Verification items for the finished model (mm, model axes). A direction names the side the tool comes from. Round coordinates to 2 decimals unless told otherwise and drop trailing zeros. Loops run counter-clockwise (first coordinate to the right, second up) from the corner with the lowest first, then second, coordinate; pieces in that order, holes last. Notation, with made-up numbers: (16, 22) - (24, 22) arc R23 ccw to (24, 54) - close; hole circle Ø9 at (13.25, 55.5). An arc over 180 degrees is marked (long way). Use CSV: the item, a comma, the result in double quotes.
```python
from build123d import *

# Parameters (mm, degrees)
F0_R          = 3
F0_R_2        = 2.5
F1_DEPTH      = 115.678
F2_R          = 2
F3_R          = 7
F6_DEPTH      = 30
F6_DEPTH_BACK = 30
F7_W          = 131.1645284295
F7_H          = 50.7057756186
F8_DEPTH      = 30
F8_DEPTH_BACK = 30


# Not quite as in the source:
# - a feature names something its author has since deleted; it is built from what else it names


with BuildPart() as f1:
    # F0 (on Top) → F1 (new body)
    with BuildSketch(Plane.XY):
        with BuildLine():
            Line((18.15, -30), (30, -30))
            Line((30, -30), (30, -18.15))
            Line((30, -18.15), (27.5, -18.15))
            Line((27.5, -18.15), (27.5, -20.15))
            Line((27.5, -20.15), (21.5477069044, -20.15))
            ThreePointArc((21.5477069044, -20.15), (19.5, -15), (21.5477069044, -9.85))
            Line((21.5477069044, -9.85), (27.5, -9.85))
            Line((27.5, -9.85), (27.5, -11.85))
            Line((27.5, -11.85), (30, -11.85))
            Line((30, -11.85), (30, 11.85))
            Line((30, 11.85), (27.5, 11.85))
            Line((27.5, 11.85), (27.5, 9.85))
            Line((27.5, 9.85), (21.5477069044, 9.85))
            ThreePointArc((21.5477069044, 9.85), (19.5, 15), (21.5477069044, 20.15))
            Line((21.5477069044, 20.15), (27.5, 20.15))
            Line((27.5, 20.15), (27.5, 18.15))
            Line((27.5, 18.15), (30, 18.15))
            Line((30, 18.15), (30, 30))
            Line((30, 30), (18.15, 30))
            Line((18.15, 30), (18.15, 27.5))
            Line((18.15, 27.5), (20.15, 27.5))
            Line((20.15, 27.5), (20.15, 21.5477069044))
            ThreePointArc((20.15, 21.5477069044), (15, 19.5), (9.85, 21.5477069044))
            Line((9.85, 21.5477069044), (9.85, 27.5))
            Line((9.85, 27.5), (11.85, 27.5))
            Line((11.85, 27.5), (11.85, 30))
            Line((11.85, 30), (-11.85, 30))
            Line((-11.85, 30), (-11.85, 27.5))
            Line((-11.85, 27.5), (-9.85, 27.5))
            Line((-9.85, 27.5), (-9.85, 21.5477069044))
            ThreePointArc((-9.85, 21.5477069044), (-15, 19.5), (-20.15, 21.5477069044))
            Line((-20.15, 21.5477069044), (-20.15, 27.5))
            Line((-20.15, 27.5), (-18.15, 27.5))
            Line((-18.15, 27.5), (-18.15, 30))
            Line((-18.15, 30), (-30, 30))
            Line((-30, 30), (-30, 18.15))
            Line((-30, 18.15), (-27.5, 18.15))
            Line((-27.5, 18.15), (-27.5, 20.15))
            Line((-27.5, 20.15), (-21.5477069044, 20.15))
            ThreePointArc((-21.5477069044, 20.15), (-19.5, 15), (-21.5477069044, 9.85))
            Line((-21.5477069044, 9.85), (-27.5, 9.85))
            Line((-27.5, 9.85), (-27.5, 11.85))
            Line((-27.5, 11.85), (-30, 11.85))
            Line((-30, 11.85), (-30, -11.85))
            Line((-30, -11.85), (-27.5, -11.85))
            Line((-27.5, -11.85), (-27.5, -9.85))
            Line((-27.5, -9.85), (-21.5477069044, -9.85))
            ThreePointArc((-21.5477069044, -9.85), (-19.5, -15), (-21.5477069044, -20.15))
            Line((-21.5477069044, -20.15), (-27.5, -20.15))
            Line((-27.5, -20.15), (-27.5, -18.15))
            Line((-27.5, -18.15), (-30, -18.15))
            Line((-30, -18.15), (-30, -30))
            Line((-30, -30), (-18.15, -30))
            Line((-18.15, -30), (-18.15, -27.5))
            Line((-18.15, -27.5), (-20.15, -27.5))
            Line((-20.15, -27.5), (-20.15, -21.5477069044))
            ThreePointArc((-20.15, -21.5477069044), (-15, -19.5), (-9.85, -21.5477069044))
            Line((-9.85, -21.5477069044), (-9.85, -27.5))
            Line((-9.85, -27.5), (-11.85, -27.5))
            Line((-11.85, -27.5), (-11.85, -30))
            Line((-11.85, -30), (11.85, -30))
            Line((11.85, -30), (11.85, -27.5))
            Line((11.85, -27.5), (9.85, -27.5))
            Line((9.85, -27.5), (9.85, -21.5477069044))
            ThreePointArc((9.85, -21.5477069044), (15, -19.5), (20.15, -21.5477069044))
            Line((20.15, -21.5477069044), (20.15, -27.5))
            Line((20.15, -27.5), (18.15, -27.5))
            Line((18.15, -27.5), (18.15, -30))
        make_face()
        with Locations((-25, -25)):
            Circle(F0_R, mode=Mode.SUBTRACT)
        with Locations((-15, -15)):
            Circle(F0_R_2, mode=Mode.SUBTRACT)
        with Locations((25, -25)):
            Circle(F0_R, mode=Mode.SUBTRACT)
        with Locations((15, -15)):
            Circle(F0_R_2, mode=Mode.SUBTRACT)
        with Locations((-25, 25)):
            Circle(F0_R, mode=Mode.SUBTRACT)
        with Locations((-15, 15)):
            Circle(F0_R_2, mode=Mode.SUBTRACT)
        Polygon((-7, 22), (-7, 27.5), (0, 27.5), (7, 27.5), (7, 22), (10, 16), (10, 10), (16, 10), (22, 7), (27.5, 7), (27.5, 0), (27.5, -7), (22, -7), (16, -10), (10, -10), (10, -16), (7, -22), (7, -27.5), (0, -27.5), (-7, -27.5), (-7, -22), (-10, -16), (-10, -10), (-16, -10), (-22, -7), (-27.5, -7), (-27.5, 0), (-27.5, 7), (-22, 7), (-16, 10), (-10, 10), (-10, 16), align=None, mode=Mode.SUBTRACT)
        with Locations((15, 15)):
            Circle(F0_R_2, mode=Mode.SUBTRACT)
        with Locations((25, 25)):
            Circle(F0_R, mode=Mode.SUBTRACT)
    extrude(amount=F1_DEPTH)

    # F2
    f2_edges = [f1.edges().sort_by_distance(p)[0] for p in [
        (-7, 27.5, 57.839),
        (7, 27.5, 57.839),
    ]]
    fillet(f2_edges, radius=F2_R)

    # F3
    f3_edges = [f1.edges().sort_by_distance(p)[0] for p in [
        (-10, 16, 57.839),
        (10, 16, 57.839),
    ]]
    fillet(f3_edges, radius=F3_R)

    # F5 (on Right) → F6 (cut, two sides)
    with BuildSketch(Plane.YZ) as f6_sk:
        Polygon((214.5999793503, -135.2321386172), (130.9673605882, 66.674863855), (-30, 0), (53.6326187621, -201.9070024722), align=None)
        Polygon((30, 115.678), (-2.0081647111, 192.9525453523), (-162.3392477394, 126.541236292), (-130.3310830283, 49.2666909397), align=None)
    extrude(amount=-F6_DEPTH, mode=Mode.SUBTRACT)
    extrude(f6_sk.sketch, amount=F6_DEPTH_BACK, mode=Mode.SUBTRACT)

    # F7 (on Right) → F8 (cut, two sides)
    with BuildSketch(Plane.YZ) as f8_sk:
        with Locations((35.5822642148, 116.1780740669)):
            Rectangle(F7_W, F7_H)
    extrude(amount=F8_DEPTH, mode=Mode.SUBTRACT)
    extrude(f8_sk.sketch, amount=-F8_DEPTH_BACK, mode=Mode.SUBTRACT)


solid = f1.part
```
1) Thickness scan on probe 1 along Y at (x, z) = (25, 40); probe 2 along Y at (x, z) = (15, 24). Record the ranges inside material, lowest first. Write a range as [from, to].
Returned:
probe 1,"y = [-30, -28], [-22, -20.15], [-9.85, -7], [7, 9.85], [20.15, 22], [28, 30]"
probe 2,"y = [-19.5, -17.5], [-12.5, -10], [10, 12.5], [17.5, 19.5]"
2) Cross-section at D-D, the plane x = -25. Record the cut outline in (y, z).
Returned:
outline,"(-30, 0) - (-28, 0.83) - (-28, 90.83) - (-30, 90.83) - close; (-22, 3.31) - (-20.15, 4.08) - (-20.15, 90.83) - (-22, 90.83) - close; (-9.85, 8.35) - (-7, 9.53) - (-7, 90.83) - (-9.85, 90.83) - close; (7, 15.33) - (9.85, 16.51) - (9.85, 90.83) - (7, 90.83) - close; (20.15, 20.77) - (22, 21.54) - (22, 90.83) - (20.15, 90.83) - close; (28, 24.02) - (30, 24.85) - (30, 90.83) - (28, 90.83) - close"
3) Gauge pin test, flat end, axial feed: pin 1 Ø2 at (x, y) = (-8, -18) entering from -Z. Record the tip position at first contact, or that the pin passes through.
Returned:
pin 1,"stops at z = 4.64"
4) Cross-section at A-A, the plane x = 4. Record the cut outline in (y, z), then the cut area to 3 significant figures.
Returned:
outline,"(-30, 0) - (-27.5, 1.04) - (-27.5, 90.83) - (-30, 90.83) - close; (27.5, 23.82) - (30, 24.85) - (30, 90.83) - (27.5, 90.83) - close"
area,"392 mm²"
5) Mould release check, pull along X, two halves, no side actions. Record for faces 1 (the face through (-30, 24, 55)), 2 (the face through (7, 24, 56)), 3 (the face through (-29, -11.85, 49)): +X half, -X half, draft (parallel to the pull), parting line (faces both ways), or undercut.
Returned:
face 1,"-X half"
face 2,"undercut"
face 3,"draft"
6) Cross-section at C-C, the plane y = 23.5. Record the cut outline in (x, z).
Returned:
outline,"(-30, 22.16) - (-27.6, 22.16) - (-27.6, 90.83) - (-30, 90.83) - close; (-22.4, 22.16) - (-20.15, 22.16) - (-20.15, 90.83) - (-22.4, 90.83) - close; (-9.85, 22.16) - (-7, 22.16) - (-7, 90.83) - (-9.85, 90.83) - close; (7, 22.16) - (9.85, 22.16) - (9.85, 90.83) - (7, 90.83) - close; (20.15, 22.16) - (22.4, 22.16) - (22.4, 90.83) - (20.15, 90.83) - close; (27.6, 22.16) - (30, 22.16) - (30, 90.83) - (27.6, 90.83) - close"
7) Access from +Z, -Z, +X, -X, +Y, -Y to the whole of each face (thin tool, end or side, straight path). Record for faces 4 (the face through (11.85, 29, 57)), 5 (the face through (-29, -18.15, 47)), 6 (the face through (-11, 27.5, 57)).
Returned:
face 4,"+Z, -Z, +Y"
face 5,"+Z, -Z, -X"
face 6,"+Z, -Z"
8) Cross-section at B-B, the plane y = 1. Record the cut outline in (x, z).
Returned:
outline,"(-30, 12.84) - (-27.5, 12.84) - (-27.5, 90.83) - (-30, 90.83) - close; (27.5, 12.84) - (30, 12.84) - (30, 90.83) - (27.5, 90.83) - close"
